Here's the drawing with two shaded views (mm, measured from the low corner). I have some questions. A direction names the side the tool comes from. Give positions to 0.01 mm unless a question says otherwise; leave off trailing zeros. Order: outer loops, then holes, each group sorted by start corner. A loop starts at its lowest first (then second) coordinate and runs counter-clockwise, first axis right, second up. Notation, with made-up numbers: (1, -15) - (15, -15) arc R11 ccw to (15, -6) - close; hole circle Ø2 at (-12, 61.25). An arc over 180 degrees is marked (long way). Use one line per item in the form item = value. Start each with the question number.
1) We'd pull the mould along Y, two halves only. Please class the marked faces 1, 2 and 3: released by +Y, released by -Y, zero draft, split by the parting line, or undercut.
2) Suppose I cut it at A-A, the plane x = 7.5. Write out the boundary of the cut face in (y, z).
3) For pin 1 (4 mm diameter, centred on y = 10, z = 5.5, fed in from -X); pin 2 (4 mm diameter, centred on x = 8, y = 7, fed in from +Z); pin 3 (1 mm diameter, centred on x = 4.5, z = 3.5, fed in from -Y), each with a flat end and sliding along its axis, tell me the tip position at first contact or that it passes through.
4) Suppose I cut it at C-C, the plane z = 14.75. Write out the boundary of the cut face in (x, y).
5) Which directions (+Z, -Z, +X, -X, +Y, -Y) give clear straight access to the entire face, cutting with the end or side of a thin tool? Please do the marked faces 4 and 5.
6) Suppose I cut it at D-D, the plane y = 10.75. Write out the boundary of the cut face in (x, z), and give its area (3 significant figures).
7) Please list where these lines run through material, in increasing order: probe 1 along Y at (x, z) = (7.5, 4.75); probe 2 along Z at (x, y) = (10, 8); probe 3 along Z at (x, y) = (5, 5).
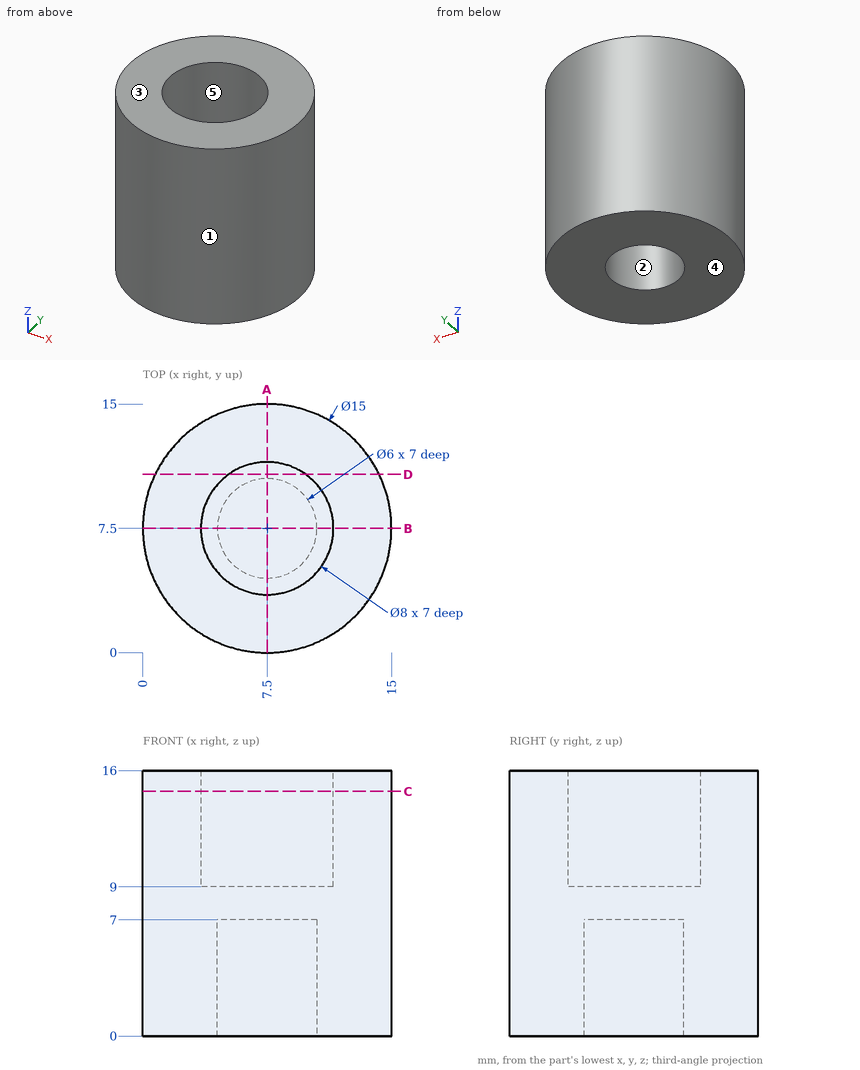
Result sheet:
q1.face_1 = split by the parting line
q1.face_2 = undercut
q1.face_3 = zero draft
q2.outline = (0, 0) - (4.5, 0) - (4.5, 7) - (10.5, 7) - (10.5, 0) - (15, 0) - (15, 16) - (11.5, 16) - (11.5, 9) - (3.5, 9) - (3.5, 16) - (0, 16) - close
q3.pin_1 = 0.02
q3.pin_2 = 9
q3.pin_3 = 0.43
q4.outline = circle Ø15 at (7.5, 7.5); hole circle Ø8 at (7.5, 7.5)
q5.face_4 = -Z, +X, -X, +Y, -Y
q5.face_5 = +Z
q6.outline = (0.74, 0) - (14.26, 0) - (14.26, 16) - (9.83, 16) - (9.83, 9) - (5.17, 9) - (5.17, 16) - (0.74, 16) - close
q6.area = 184 mm²
q7.probe_1 = 0 to 4.5, 10.5 to 15
q7.probe_2 = 7 to 9
q7.probe_3 = 0 to 9
